Part model, mm, in its own coordinate system. Give positions to 0.01 mm unless a question says otherwise; leave off trailing zeros. Order: outer loops, then holes, each group sorted by start corner. A loop starts at its lowest first (then second) coordinate and runs counter-clockwise, first axis right, second up. Notation, with made-up numbers: M -1.75,39 L 22.25,39 A18 cw 22.25,74 Z; hole C 42,80.25 d10. An arc over 180 degrees is marked long. Return JSON: item names as keys, results as strings.
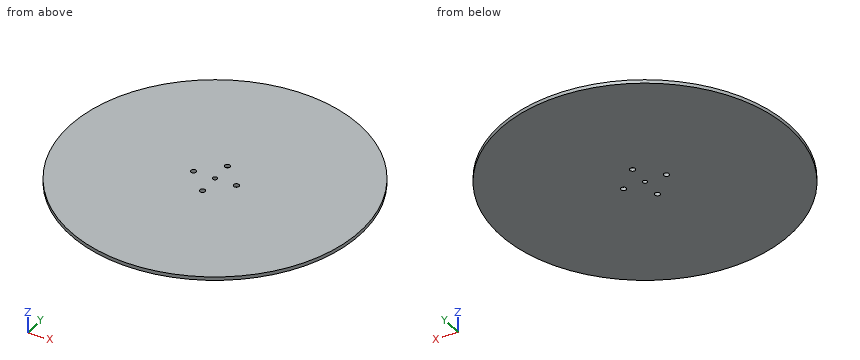
from build123d import *

# Parameters (mm, degrees)
F0_R     = 165
F0_R_2   = 3
F0_R_3   = 2.5
F1_DEPTH = 4


with BuildPart() as f1:
    # F0 (on Top) → F1 (new body)
    with BuildSketch(Plane.XY):
        with Locations((140.095845, 209.353372)):
            Circle(F0_R)
        with Locations((140.095845, 185.586029)):
            Circle(F0_R_2, mode=Mode.SUBTRACT)
        with Locations((116.328501, 209.353372)):
            Circle(F0_R_2, mode=Mode.SUBTRACT)
        with Locations((140.095845, 209.353372)):
            Circle(F0_R_3, mode=Mode.SUBTRACT)
        with Locations((163.863189, 209.353372)):
            Circle(F0_R_2, mode=Mode.SUBTRACT)
        with Locations((140.095845, 233.120716)):
            Circle(F0_R_2, mode=Mode.SUBTRACT)
    extrude(amount=F1_DEPTH)


solid = f1.part
Q1. Band-saw the part on A-A (z = 2.5). Give the cut face in (x, y), then the cut area to 3 significant figures.
Established:
{"outline": "C 140.1,209.35 d330; hole C 116.33,209.35 d6; hole C 140.1,185.59 d6; hole C 140.1,233.12 d6; hole C 140.1,209.35 d5; hole C 163.86,209.35 d6", "area": "85,400 mm²"}
Q2. Band-saw the part on B-B (y = 89). Give the cut face in (x, z), then the cut area to 3 significant figures.
Established:
{"outline": "M 27.22,0 L 252.97,0 L 252.97,4 L 27.22,4 Z", "area": "903 mm²"}
Q3. Pin check, flat tips, straight feed: pin 1 (4 mm diameter, centred on x = 140.1, y = 209.35, fed in from +Z); pin 2 (1.5 mm diameter, centred on y = 241, z = 1, fed in from -X); pin 3 (1 mm diameter, centred on x = 30.5, y = 184, fed in from -Z); pin 4 (1.5 mm diameter, centred on x = 14.5, z = 1, fed in from +Y). Stop position of each tip, or through.
Established:
{"pin 1": "passes through", "pin 2": "stops at x = -21.99", "pin 3": "stops at z = 0", "pin 4": "stops at y = 317.24"}
Q4. Probe line 1 along Y through (x, z) = (141, 2.95); line 2 along Y through (x, z) = (166.5, 0.55); line 3 along Y through (x, z) = (142, 1.3). List the from-to ranges inside material, lowest first.
Established:
{"line 1": "y = 44.36 to 182.73, 188.45 to 207.02, 211.68 to 230.26, 235.98 to 374.35", "line 2": "y = 46.48 to 207.92, 210.78 to 372.23", "line 3": "y = 44.36 to 183.27, 187.9 to 207.73, 210.97 to 230.8, 235.44 to 374.34"}
Q5. Band-saw the part on C-C (x = 61.5). Give the cut face in (y, z).
Established:
{"outline": "M 64.28,0 L 354.43,0 L 354.43,4 L 64.28,4 Z"}
